Part model, mm, in its own coordinate system. A direction names the side the tool comes from. Coordinates: 2 decimals unless noted, no trailing zeros. Write each loop counter-clockwise with the first axis right and the second up, starting at its lowest first coordinate (ties: lowest second). Pieces come first, ordered by that corner, then holes. Notation, with made-up numbers: (64.5, 78.25) - (116.5, 78.25) arc R20 cw to (116.5, 113.25) - close; hole circle Ø3 at (21, -9.5). An arc over 180 degrees is marked (long way). Use a Markdown table: item, result.
```python
from build123d import *

# Parameters (mm, degrees)
F5_DEPTH = 26


with BuildPart() as f1:
    # F0 (on Front) → F1 (revolve)
    with BuildSketch(Plane.XZ):
        Polygon((0, 0), (-8, 0), (-8, -3.7), (-6, -3.7), (-6, -9.7), (-8, -9.7), (-8, -12.7), (-8, -16.7), (-11.15, -16.7), (-11.15, -42.7), (0, -42.7), align=None)
    revolve(axis=Axis((0, 0, -21.35), (0, 0, -1)))

    # F2 (on Front) → F3 (revolve)
    with BuildSketch(Plane.XZ):
        Polygon((0, -62.3), (0, -42.7), (-3.5, -42.7), (-3.5, -58.8), align=None)
    revolve(axis=Axis((0, 0, -52.5), (0, 0, 1)))

    # F4 (on face) → F5 (join, through all)
    with BuildSketch(Plane(origin=(0, 0, -42.7), x_dir=(1, 0, 0), z_dir=(0, 0, -1))):
        with BuildLine():
            ThreePointArc((0, 11.15), (11.15, 0), (0, -11.15))
            Line((0, -11.15), (25, -15))
            Line((25, -15), (25, 15))
            Line((25, 15), (0, 11.15))
        make_face()
    extrude(amount=-F5_DEPTH)


solid = f1.part
```
Item 1: Band-saw the part on C-C, the plane z = -15.5. Give the cut face in (x, y).
From the geometry:
| item | result |
|---|---|
| outline | circle Ø16 at (0, 0) |
Item 2: Two-plate mould, pull along Z, no slides. Class faces 4 (the face through (0.205, 0.925, -61.352)), 5 (the face through (2, 6, -3.7)), 6 (the face through (25, 0, -30)): pulls with the +Z half, pulls with the -Z half, needs draft (parallel to the pull), parting line crosses it, or undercut.
From the geometry:
| item | result |
|---|---|
| face 4 | pulls with the -Z half |
| face 5 | undercut |
| face 6 | needs draft |
Item 3: Band-saw the part on B-B, the plane x = 5. Give the cut face in (y, z) (3 decimals).
From the geometry:
| item | result |
|---|---|
| outline | (-11.92, -42.7) - (11.92, -42.7) - (11.92, -16.7) - (6.245, -16.7) - (6.245, -9.7) - (3.317, -9.7) - (3.317, -3.7) - (6.245, -3.7) - (6.245, 0) - (-6.245, 0) - (-6.245, -3.7) - (-3.317, -3.7) - (-3.317, -9.7) - (-6.245, -9.7) - (-6.245, -16.7) - (-11.92, -16.7) - close |
Item 4: Drop flat-ended pins along their axis: P1, Ø8, axis at y = -4.5, z = -9, coming from the -X side; P2, Ø10, axis at x = 15, y = -2.5, coming from the +Z side; P3, Ø9, axis at x = 0, y = -5, coming from the -Z side. Give the stop position or say it passes through.
From the geometry:
| item | result |
|---|---|
| P1 | x = -7.98 |
| P2 | z = -16.7 |
| P3 | z = -61.8 |
Item 5: Drill centre lines: probe 1 along Z at (x, y) = (21, -10); probe 2 along X at (y, z) = (-0.25, -54.5); probe 3 along Z at (x, y) = (7.5, -1.5). Where is each one in solid material? Low to high.
From the geometry:
| item | result |
|---|---|
| probe 1 | -42.7 to -16.7 |
| probe 2 | -3.49 to 3.49 |
| probe 3 | -42.7 to -9.7, -3.7 to 0 |
Item 6: Band-saw the part on D-D, the plane y = -7. Give the cut face in (x, z).
From the geometry:
| item | result |
|---|---|
| outline | (-8.68, -42.7) - (25, -42.7) - (25, -16.7) - (3.87, -16.7) - (3.87, -9.7) - (-3.87, -9.7) - (-3.87, -16.7) - (-8.68, -16.7) - close; (-3.87, -3.7) - (3.87, -3.7) - (3.87, 0) - (-3.87, 0) - close |
Item 7: Band-saw the part on A-A, the plane y = 6.75. Give the cut face in (x, z).
From the geometry:
| item | result |
|---|---|
| outline | (-8.87, -42.7) - (25, -42.7) - (25, -16.7) - (4.29, -16.7) - (4.29, -9.7) - (-4.29, -9.7) - (-4.29, -16.7) - (-8.87, -16.7) - close; (-4.29, -3.7) - (4.29, -3.7) - (4.29, 0) - (-4.29, 0) - close |
Item 8: Which spindle directions (+Z, -Z, +X, -X, +Y, -Y) get a long thin tool onto all of the face, cutting with end or side? Do faces 1 (the face through (-3.233, 1.341, -50.863)), 2 (the face through (-2, 6, -9.7)), 3 (the face through (1.73, -7.81, -1.88)). Say none if no direction does.
From the geometry:
| item | result |
|---|---|
| face 1 | -Z |
| face 2 | none |
| face 3 | +Z |
